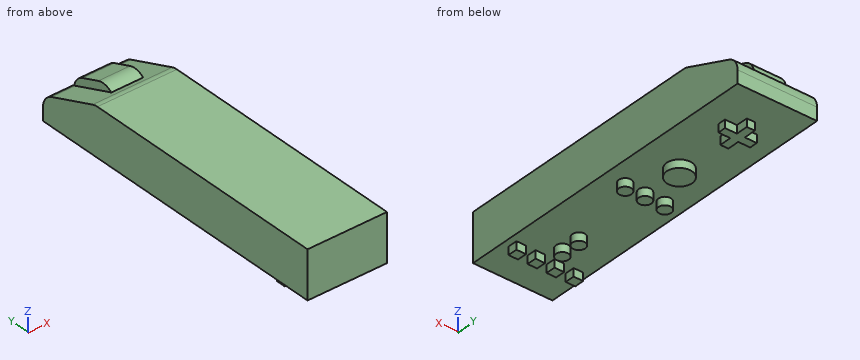
from build123d import *

# Parameters (mm, degrees)
CROQUIS1_W              = 50
CROQUIS1_H              = 200
SALIENTE_EXTRUIR1_DEPTH = 30
CORTAR_EXTRUIR1_DEPTH   = 60
CROQUIS3_W              = 20
CROQUIS3_H              = 30
SALIENTE_EXTRUIR2_DEPTH = 5
REDONDEO1_R             = 10
REDONDEO2_R             = 10
CROQUIS5_W              = 6
CROQUIS5_H              = 6
CROQUIS5_R              = 8
CROQUIS5_R_2            = 4
SALIENTE_EXTRUIR3_DEPTH = 5


with BuildPart() as part:
    # Croquis1 → Saliente-Extruir1 (new body)
    with BuildSketch(Plane.XY):
        Rectangle(CROQUIS1_W, CROQUIS1_H)
    extrude(amount=SALIENTE_EXTRUIR1_DEPTH)

    # Croquis2 → Cortar-Extruir1 (cut)
    with BuildSketch(Plane.ZY.offset(25)):
        Polygon((15, 100), (30, 60.706463385), (30, 100), align=None)
    extrude(amount=-CORTAR_EXTRUIR1_DEPTH, mode=Mode.SUBTRACT)

    # Croquis3 → Saliente-Extruir2 (add)
    with BuildSketch(Plane(origin=(0, 17.716995079, 46.41089299), x_dir=(1, 0, 0), z_dir=(0, 0.356639588239418, 0.9342420479192843))):
        with Locations((0, 67.044976998)):
            Rectangle(CROQUIS3_W, CROQUIS3_H)
    extrude(amount=SALIENTE_EXTRUIR2_DEPTH)

    # Redondeo1
    # the kernel refuses this fillet: 10 mm, written as the material it takes off along each edge
    with BuildSketch(Plane(origin=(-29.60955221, 60.706463385, 30), x_dir=(0, -1, 0), z_dir=(1, 0, 0))) as redondeo1_piece_1:
        with BuildLine():
            CenterArc((REDONDEO1_R * 0.184382088386, REDONDEO1_R), REDONDEO1_R, 249.106035538, 20.893964462)
            Line((-REDONDEO1_R * 0.172257499853, REDONDEO1_R * 0.0657579520807), (0, 0))
            Line((0, 0), (REDONDEO1_R * 0.184382088386, 0))
        make_face()
    extrude(amount=59.219104419, mode=Mode.SUBTRACT)
    with BuildSketch(Plane(origin=(-42.216106179, 100, 15), x_dir=(0, -0.934242047919284, 0.3566395882394187), z_dir=(1, 0, 0))) as redondeo1_piece_2_section:
        with BuildLine():
            CenterArc((REDONDEO1_R * 0.688644247166, REDONDEO1_R), REDONDEO1_R, 200.893964462, 69.106035538)
            Line((-REDONDEO1_R * 0.245597800753, REDONDEO1_R * 0.643360411761), (0, 0))
            Line((0, 0), (REDONDEO1_R * 0.688644247166, 0))
        make_face()
    redondeo1_piece_2 = extrude(amount=84.432212358, mode=Mode.PRIVATE)
    redondeo1_piece_2 = split(redondeo1_piece_2, bisect_by=Plane(origin=(-10, 94.011560914, 17.386219939), z_dir=(-1, 0, 0)), keep=Keep.TOP, mode=Mode.PRIVATE)
    redondeo1_piece_2 = split(redondeo1_piece_2, bisect_by=Plane(origin=(-26.10805309, 94.400241221, 17.237844274), z_dir=(0, -0.9342420479192843, 0.35663958823941805)), keep=Keep.TOP, mode=Mode.PRIVATE)
    add(redondeo1_piece_2, mode=Mode.SUBTRACT)
    with BuildSketch(Plane(origin=(-42.216106179, 100, 15), x_dir=(0, -0.934242047919284, 0.3566395882394187), z_dir=(1, 0, 0))) as redondeo1_piece_3_section:
        with BuildLine():
            CenterArc((REDONDEO1_R * 0.688644247166, REDONDEO1_R), REDONDEO1_R, 200.893964462, 69.106035538)
            Line((-REDONDEO1_R * 0.245597800753, REDONDEO1_R * 0.643360411761), (0, 0))
            Line((0, 0), (REDONDEO1_R * 0.688644247166, 0))
        make_face()
    redondeo1_piece_3 = extrude(amount=84.432212358, mode=Mode.PRIVATE)
    redondeo1_piece_3 = split(redondeo1_piece_3, bisect_by=Plane(origin=(-10, 98.665500542, 13.974903393), z_dir=(-1, 0, 0)), keep=Keep.TOP, mode=Mode.PRIVATE)
    redondeo1_piece_3 = split(redondeo1_piece_3, bisect_by=Plane(origin=(-26.10805309, 93.855575449, 15.811054644), z_dir=(0, 0.9342420479192843, -0.35663958823941805)), keep=Keep.TOP, mode=Mode.PRIVATE)
    add(redondeo1_piece_3, mode=Mode.SUBTRACT)
    with BuildSketch(Plane(origin=(-42.216106179, 100, 15), x_dir=(0, -0.934242047919284, 0.3566395882394187), z_dir=(1, 0, 0))) as redondeo1_piece_4_section:
        with BuildLine():
            CenterArc((REDONDEO1_R * 0.688644247166, REDONDEO1_R), REDONDEO1_R, 200.893964462, 69.106035538)
            Line((-REDONDEO1_R * 0.245597800753, REDONDEO1_R * 0.643360411761), (0, 0))
            Line((0, 0), (REDONDEO1_R * 0.688644247166, 0))
        make_face()
    redondeo1_piece_4 = extrude(amount=84.432212358, mode=Mode.PRIVATE)
    redondeo1_piece_4 = split(redondeo1_piece_4, bisect_by=Plane(origin=(-10, 98.665500542, 13.974903393), z_dir=(1, 0, 0)), keep=Keep.TOP, mode=Mode.PRIVATE)
    redondeo1_piece_4 = split(redondeo1_piece_4, bisect_by=Plane(origin=(0, 93.855575449, 15.811054644), z_dir=(0, 0.9342420479192843, -0.35663958823941805)), keep=Keep.TOP, mode=Mode.PRIVATE)
    redondeo1_piece_4 = split(redondeo1_piece_4, bisect_by=Plane(origin=(10, 98.665500542, 13.974903393), z_dir=(-1, 0, 0)), keep=Keep.TOP, mode=Mode.PRIVATE)
    add(redondeo1_piece_4, mode=Mode.SUBTRACT)
    with BuildSketch(Plane(origin=(-42.216106179, 100, 15), x_dir=(0, -0.934242047919284, 0.3566395882394187), z_dir=(1, 0, 0))) as redondeo1_piece_5_section:
        with BuildLine():
            CenterArc((REDONDEO1_R * 0.688644247166, REDONDEO1_R), REDONDEO1_R, 200.893964462, 69.106035538)
            Line((-REDONDEO1_R * 0.245597800753, REDONDEO1_R * 0.643360411761), (0, 0))
            Line((0, 0), (REDONDEO1_R * 0.688644247166, 0))
        make_face()
    redondeo1_piece_5 = extrude(amount=84.432212358, mode=Mode.PRIVATE)
    redondeo1_piece_5 = split(redondeo1_piece_5, bisect_by=Plane(origin=(26.10805309, 94.400241221, 17.237844274), z_dir=(0, -0.9342420479192843, 0.35663958823941805)), keep=Keep.TOP, mode=Mode.PRIVATE)
    redondeo1_piece_5 = split(redondeo1_piece_5, bisect_by=Plane(origin=(10, 94.011560914, 17.386219939), z_dir=(1, 0, 0)), keep=Keep.TOP, mode=Mode.PRIVATE)
    add(redondeo1_piece_5, mode=Mode.SUBTRACT)
    with BuildSketch(Plane(origin=(-42.216106179, 100, 15), x_dir=(0, -0.934242047919284, 0.3566395882394187), z_dir=(1, 0, 0))) as redondeo1_piece_6_section:
        with BuildLine():
            CenterArc((REDONDEO1_R * 0.688644247166, REDONDEO1_R), REDONDEO1_R, 200.893964462, 69.106035538)
            Line((-REDONDEO1_R * 0.245597800753, REDONDEO1_R * 0.643360411761), (0, 0))
            Line((0, 0), (REDONDEO1_R * 0.688644247166, 0))
        make_face()
    redondeo1_piece_6 = extrude(amount=84.432212358, mode=Mode.PRIVATE)
    redondeo1_piece_6 = split(redondeo1_piece_6, bisect_by=Plane(origin=(26.10805309, 93.855575449, 15.811054644), z_dir=(0, 0.9342420479192843, -0.35663958823941805)), keep=Keep.TOP, mode=Mode.PRIVATE)
    redondeo1_piece_6 = split(redondeo1_piece_6, bisect_by=Plane(origin=(10, 98.665500542, 13.974903393), z_dir=(1, 0, 0)), keep=Keep.TOP, mode=Mode.PRIVATE)
    add(redondeo1_piece_6, mode=Mode.SUBTRACT)

    # Redondeo2
    # the kernel refuses this fillet: 10 mm, written as the material it takes off along each edge
    with BuildSketch(Plane(origin=(31.650635095, 68.122798915, 32.520804063), x_dir=(0, 0.9342420479192848, -0.3566395882394171), z_dir=(-1, 0, 0))) as redondeo2_piece_1:
        with BuildLine():
            CenterArc((8.660254038, 10), REDONDEO2_R, 210, 60)
            Line((0, 5), (-0.173205081, 4.9))
            ThreePointArc((-0.173205081, 4.9), (-0.2, 2.5), (-0.2, 0))
            Line((-0.2, 0), (0, -0.2))
            Line((0, -0.2), (8.660254038, -0.2))
            Line((8.660254038, -0.2), (8.660254038, 0))
        make_face()
    extrude(amount=63.301270189, mode=Mode.SUBTRACT)
    with BuildSketch(Plane(origin=(-31.703453679, 96.150060353, 21.821616416), x_dir=(0, -0.3566395882395135, -0.9342420479192478), z_dir=(1, 0, 0))) as redondeo2_piece_2:
        with BuildLine():
            CenterArc((10, -8.681381471), REDONDEO2_R, 119.757004223, 60.242995777)
            Line((0, -8.681381471), (-0.2, -8.681381471))
            Line((-0.2, -8.681381471), (-0.2, 0))
            Line((-0.2, 0), (0, 0.2))
            ThreePointArc((0, 0.2), (2.518386828, 0.2), (4.937509129, 0.173627629))
            Line((4.937509129, 0.173627629), (5.036773655, 0))
        make_face()
    extrude(amount=63.406907357, mode=Mode.SUBTRACT)

    # Croquis5 → Saliente-Extruir3 (add)
    with BuildSketch(Plane(origin=(0, 0, 0), x_dir=(-1, 0, 0), z_dir=(0, 0, -1))):
        Polygon((-2.5, 80), (-2.5, 72.5), (-10, 72.5), (-10, 67.5), (-2.5, 67.5), (-2.5, 60), (2.5, 60), (2.5, 67.5), (10, 67.5), (10, 72.5), (2.5, 72.5), (2.5, 80), align=None)
        with Locations((-17.908573371, -75.072215566)):
            Rectangle(CROQUIS5_W, CROQUIS5_H)
        with Locations((18.091426629, -75.072215566)):
            Rectangle(CROQUIS5_W, CROQUIS5_H)
        with Locations((-5.908573371, -75.072215566)):
            Rectangle(CROQUIS5_W, CROQUIS5_H)
        with Locations((6.091426629, -75.072215566)):
            Rectangle(CROQUIS5_W, CROQUIS5_H)
        with Locations(Location((0, 26, 0), (0, 0, 180))):
            Circle(CROQUIS5_R)
        with Locations(Location((0, 0, 0), (0, 0, 180))):
            Circle(CROQUIS5_R_2)
        with Locations(Location((-12.5, 0, 0), (0, 0, 180))):
            Circle(CROQUIS5_R_2)
        with Locations(Location((12.5, 0, 0), (0, 0, 180))):
            Circle(CROQUIS5_R_2)
        with Locations(Location((0, -50, 0), (0, 0, 180))):
            Circle(CROQUIS5_R_2)
        with Locations(Location((0, -62.5, 0), (0, 0, 180))):
            Circle(CROQUIS5_R_2)
    extrude(amount=SALIENTE_EXTRUIR3_DEPTH)


solid = part.part
Check sheet for the modelled part. Datum: model origin and axes. Units: mm. Round coordinates to 2 decimals unless told otherwise and drop trailing zeros. Order: outer loops, then holes, each group sorted by start corner. A loop starts at its lowest first (then second) coordinate and runs counter-clockwise, first axis right, second up. Notation, with made-up numbers: M -32.75,73 L -25.75,73 A28 ccw -25.75,94 Z; hole C -26.75,5.5 d2. An arc over 180 degrees is marked long. One line per item, written item: value. Start each with the question number.
1. Gauge pin test, flat ends, axial feed: P1, Ø2.5, axis at x = 0, z = -1.5, coming from the -Y side; P2, Ø4, axis at y = -74.5, z = -2.5, coming from the +X side; P3, Ø5.5, axis at x = 17.5, z = -3, coming from the +Y side. Record the tip position at first contact, or that the pin passes through.
2. Section check B-B on y = -62.5. Enter the section's corners in (x, z), and give its area (3 significant figures).
3. Section check D-D on z = 23. Enter the section's corners in (x, y).
4. Scan lines: line 1 along Z through (x, y) = (9, -26); line 2 along Z through (x, y) = (3.5, 31.5); line 3 along Y through (x, z) = (-5, 21). Record each from-to range of solid material in increasing order.
5. Section check A-A on z = -2. Give the number of separate pieces and of enclosed holes in the cut face, and give its area (3 significant figures).
Results found:
1. P1: y = -66.5
1. P2: x = 20.91
1. P3: y = 3.31
2. outline: M -25,0 L -4,0 L -4,-5 L 4,-5 L 4,0 L 25,0 L 25,30 L -25,30 Z
2. area: 1,540 mm^2
3. outline: M -25,-100 L 25,-100 L 25,79.04 L 10,79.04 L 10,91.17 L -10,91.17 L -10,79.04 L -25,79.04 Z
4. line 1: 0 to 30
4. line 2: -5 to 30
4. line 3: -100 to 92.87
5. separate pieces: 11
5. enclosed holes: 0
5. area: 771 mm^2
